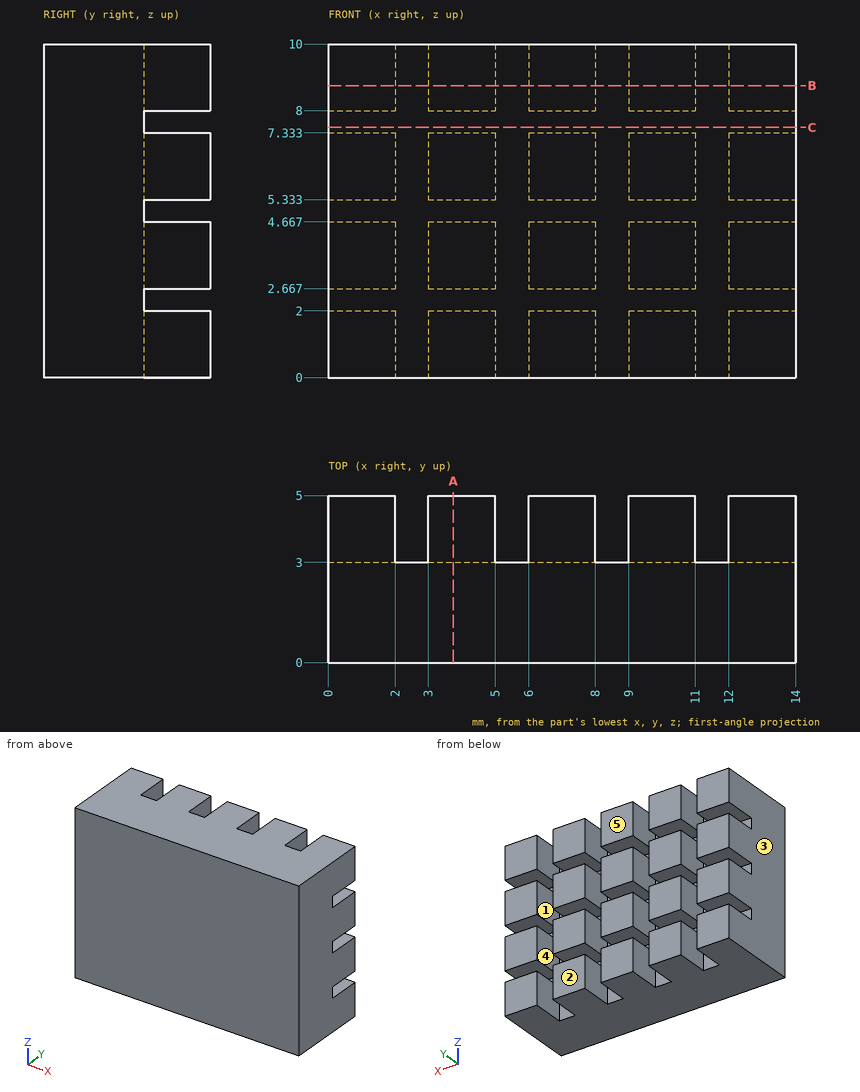
Job drawing, mm, ordinate dimensions from the low corner. One solid piece. A direction names the side the tool comes from. Coordinates: 2 decimals unless noted, no trailing zeros. Order: outer loops, then holes, each group sorted by start corner. A loop starts at its lowest first (then second) coordinate and runs counter-clockwise, first axis right, second up. Notation, with made-up numbers: (33, 26.5) - (53, 26.5) arc R14 cw to (53, 48.5) - close; hole circle Ø5 at (77, -19). An arc over 180 degrees is marked (long way). Return JSON: item names as keys, results as strings. Group by question number.
1) Mould opens along X. For the marked faces 1, 2 and 3 say: released by +X, released by -X, zero draft, split by the parting line, or undercut.
2) Saw through at C-C, the plane z = 7.5. Write the cut outline in (x, y).
3) Tool access for the marked faces 4 and 5: list every direction of +Z, -Z, +X, -X, +Y, -Y with a clear straight run to the whole face (end or side of a thin tool).
4) Saw through at A-A, the plane x = 3.75. Write the cut outline in (y, z), plus the area to 3 significant figures.
5) Saw through at B-B, the plane z = 8.75. Write the cut outline in (x, y).
6) Probe line 1 (X direction, y = 4.7, z = 1.75); line 2 (Z direction, x = 6.5, y = 3.55); line 3 (Y direction, x = 11.5, z = 4.25). List the from-to ranges inside material, lowest first. Write a range as from..to.
Values found:
{
 "1": {"face 1": "undercut", "face 2": "zero draft", "face 3": "released by -X"},
 "2": {"outline": "(0, 0) - (14, 0) - (14, 3) - (0, 3) - close"},
 "3": {"face 4": "+Z, -Z, +Y", "face 5": "+Z, -Z, +X, -X, +Y"},
 "4": {"outline": "(0, 0) - (5, 0) - (5, 2) - (3, 2) - (3, 2.67) - (5, 2.67) - (5, 4.67) - (3, 4.67) - (3, 5.33) - (5, 5.33) - (5, 7.33) - (3, 7.33) - (3, 8) - (5, 8) - (5, 10) - (0, 10) - close", "area": "46.0 mm²"},
 "5": {"outline": "(0, 0) - (14, 0) - (14, 5) - (12, 5) - (12, 3) - (11, 3) - (11, 5) - (9, 5) - (9, 3) - (8, 3) - (8, 5) - (6, 5) - (6, 3) - (5, 3) - (5, 5) - (3, 5) - (3, 3) - (2, 3) - (2, 5) - (0, 5) - close"},
 "6": {"line 1": "x = 0..2, 3..5, 6..8, 9..11, 12..14", "line 2": "z = 0..2, 2.67..4.67, 5.33..7.33, 8..10", "line 3": "y = 0..3"}
}
